Input: part model. Units: mm. Frame: model coordinates. A direction names the side the tool comes from. Round coordinates to 2 decimals unless told otherwise and drop trailing zeros. Loops run counter-clockwise (first coordinate to the right, second up) from the corner with the lowest first, then second, coordinate; pieces in that order, holes last. Notation, with made-up numbers: (55.25, 39.25) -> (89.25, 39.25) arc R10 ccw to (89.25, 46.25) -> close; hole circle Ø5 at (33, 83.5). An arc over 180 degrees is marked (long way). Answer as a JSON object with one key per item and string values. Group by question number.
Item 1: Material intervals for line 1 (Y direction, x = 0, z = 12.5); line 2 (Z direction, x = 3, y = 0), sorted ascending. Write a range as [from, to].
Item 2: Set-up query: faces 4 (the flat face through (0, 0, 0)), 5 (the cylindrical face through (6.401, 0.555, 16.339)), 6 (the cylindrical face through (-3.695, -1.532, 14.93)). Return all of +Z, -Z, +X, -X, +Y, -Y with unobstructed straight access to the full face (end or side cutting, diameter ignored); none if empty.
Item 3: Section query A-A on y = 0. Return loops of the section in (x, z).
Item 4: Pin query (flat end, axial travel): pin 1 (1.5 mm diameter, centred on x = 5, z = 15, fed in from +Y); pin 2 (5 mm diameter, centred on x = -5, z = 2.5, fed in from +Y); pin 3 (4 mm diameter, centred on y = 5, z = 4, fed in from -X). Return the tip coordinate at first contact, or that it passes through.
Item 5: Draft query along X for faces 1 (the flat face through (-3, -3, 20)), 2 (the cylindrical face through (-8.584, 2.703, 10.119)), 3 (the flat face through (0, 0, 10)). Return one class per face: released by +X, released by -X, zero draft, split by the parting line, or undercut.
Item 6: Section query C-C on z = 11.5. Return loops of the section in (x, y).
Item 7: Section query D-D on z = 3.25. Return loops of the section in (x, y).
Item 8: Section query B-B on x = 0. Return loops of the section in (y, z), and give its area (3 significant figures).
from build123d import *

# Parameters (mm, degrees)
F_8_0_8_DIAMETER_HOLE1_D     = 8
F_8_0_8_DIAMETER_HOLE1_DEPTH = 10
SKETCH4_W                    = 1.45
SKETCH4_H                    = 18


with BuildPart() as part:
    # Sketch1 → Revolve1 (revolve)
    with BuildSketch(Plane.XZ, mode=Mode.PRIVATE) as revolve1_sk:
        with BuildLine():
            Line((7.5, 20), (0, 20))
            Line((0, 20), (0, 0))
            Line((0, 0), (7.5, 0))
            ThreePointArc((7.5, 0), (8.560660172, 0.439339828), (9, 1.5))
            Line((9, 1.5), (9, 18.5))
            ThreePointArc((9, 18.5), (8.560660172, 19.560660172), (7.5, 20))
        make_face()
    revolve(revolve1_sk.sketch.rotate(Axis((0, 0, 20), (0, 0, -1)), 180), axis=Axis((0, 0, 20), (0, 0, -1)))

    # Ø8.0 (8) Diameter Hole1
    with Locations(Plane.XY.offset(20)):
        with Locations((0, 0)):
            Hole(F_8_0_8_DIAMETER_HOLE1_D / 2, depth=F_8_0_8_DIAMETER_HOLE1_DEPTH)

    # Sketch4 → Ø2.9 (2.9) Diameter Hole1 (revolve, cut)
    with BuildSketch(Plane(origin=(3.727935085, 0, 15), x_dir=(0, 0, 1), z_dir=(0, 1, 0))):
        with Locations((0.725, 9)):
            Rectangle(SKETCH4_W, SKETCH4_H)
    revolve(axis=Axis((-2.622064915, 0, 15), (1, 0, 0)), mode=Mode.SUBTRACT)


solid = part.part
Solved:
{
 "1": {"line 1": "[-9, -4], [4, 9]", "line 2": "[0, 10]"},
 "2": {"face 4": "-Z, +X, -X, +Y, -Y", "face 5": "+X", "face 6": "+Z"},
 "3": {"outline": "(-9, 1.5) arc R1.5 ccw to (-7.5, 0) -> (7.5, 0) arc R1.5 ccw to (9, 1.5) -> (9, 13.55) -> (4, 13.55) -> (4, 10) -> (-4, 10) -> (-4, 20) -> (-7.5, 20) arc R1.5 ccw to (-9, 18.5) -> close; (4, 16.45) -> (9, 16.45) -> (9, 18.5) arc R1.5 ccw to (7.5, 20) -> (4, 20) -> close"},
 "4": {"pin 1": "y = 7.93", "pin 2": "y = 8.65", "pin 3": "x = -8.49"},
 "5": {"face 1": "zero draft", "face 2": "split by the parting line", "face 3": "undercut"},
 "6": {"outline": "circle Ø18 at (0, 0); hole circle Ø8 at (0, 0)"},
 "7": {"outline": "circle Ø18 at (0, 0)"},
 "8": {"outline": "(-9, 1.5) arc R1.5 ccw to (-7.5, 0) -> (7.5, 0) arc R1.5 ccw to (9, 1.5) -> (9, 18.5) arc R1.5 ccw to (7.5, 20) -> (4, 20) -> (4, 10) -> (-4, 10) -> (-4, 20) -> (-7.5, 20) arc R1.5 ccw to (-9, 18.5) -> close", "area": "278 mm²"}
}
